Part print with two shaded views. Sizes in mm from the minimum x, y, z corner. Coordinates: 2 decimals unless noted, no trailing zeros. Loops run counter-clockwise (first coordinate to the right, second up) from the corner with the lowest first, then second, coordinate; pieces in that order, holes last.
(1) Two-plate mould, pull along X, no slides. Class the marked faces 1, 2 and 3: pulls with the +X half, pulls with the -X half, needs draft (parallel to the pull), parting line crosses it, or undercut.
(2) Slice it at A-A (x = 55.5). Give the cut face in (y, z).
(3) Wall check: L1, parallel to Y at x = 25.5, z = 16; L2, parallel to X at y = 70, z = 46; L3, parallel to Y at x = 49, z = 37. Give the ranges that are in metal, low to high.
(4) Slice it at B-B (y = 43.5). Give the cut face in (x, z).
(5) Flat gauge pins, fed straight in: P1, Ø8, axis at x = 29.5, y = 57, coming from the +Z side; P2, Ø1, axis at x = 48, z = 61.5, coming from the -Y side; P3, Ø6, axis at x = 24.5, z = 33.5, coming from the -Y side; P4, Ø12, axis at x = 24.5, y = 41.5, coming from the +Z side. Where does each tip first touch, or does it go through?
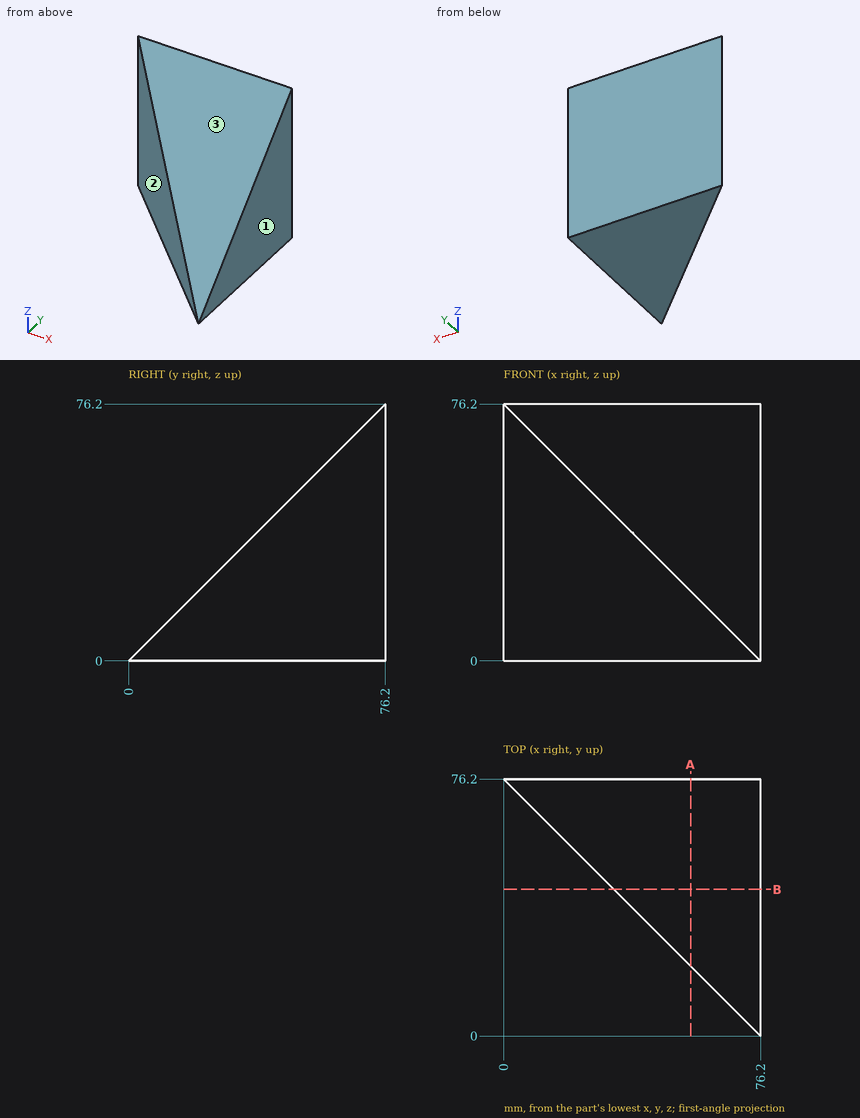
Response values:
1. face 1: pulls with the +X half
1. face 2: pulls with the -X half
1. face 3: needs draft
2. outline: (20.7, 0) - (76.2, 0) - (76.2, 76.2) - (20.7, 20.7) - close
3. L1: y = 50.7 to 76.2
3. L2: x = 6.2 to 76.2
3. L3: y = 37 to 76.2
4. outline: (32.7, 0) - (76.2, 0) - (76.2, 43.5) - (32.7, 43.5) - close
5. P1: stops at z = 61
5. P2: stops at y = 61
5. P3: stops at y = 48.7
5. P4: passes through
